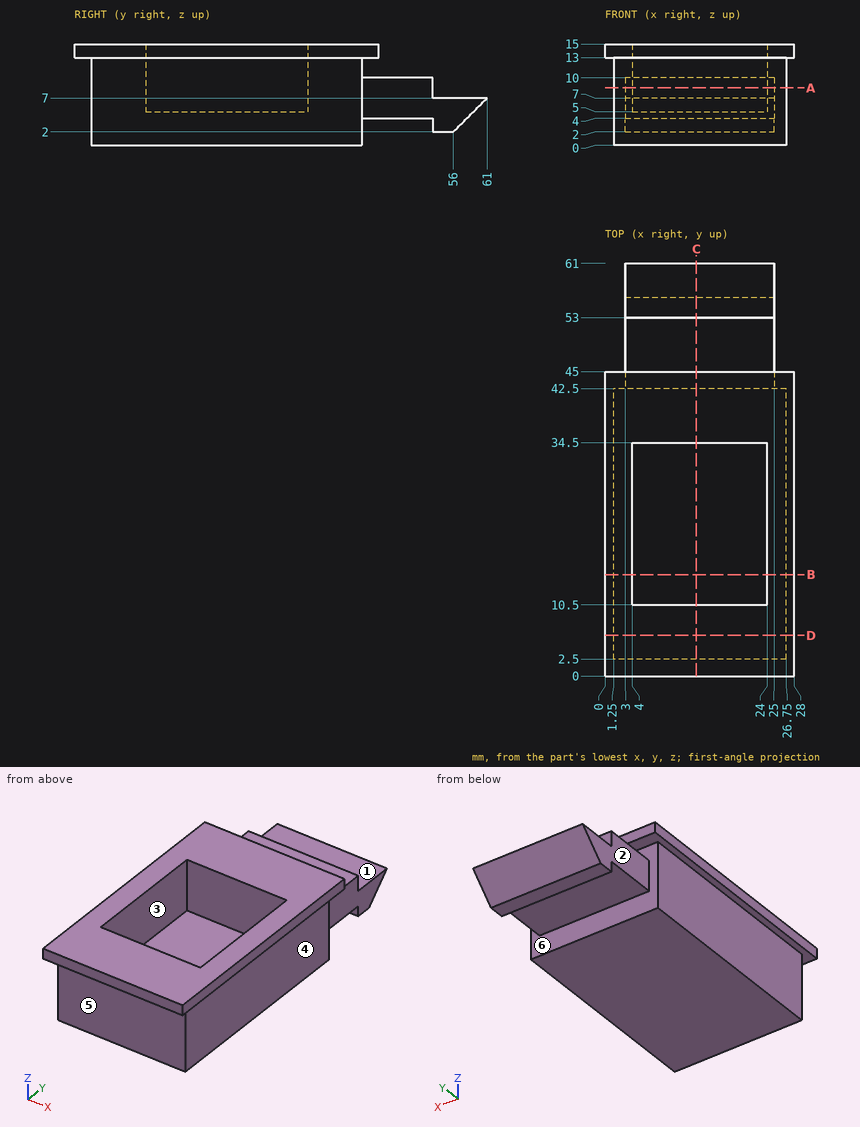
Geometry: see drawing. Coordinates: mm, zero at the bounding-box minimum. A direction names the side the tool comes from. Give positions to 0.01 mm unless a question says otherwise; leave off trailing zeros. Loops run counter-clockwise (first coordinate to the right, second up) from the corner with the lowest first, then second, coordinate; pieces in that order, holes last. Notation, with made-up numbers: M 12,-8.75 L 63,-8.75 A7 ccw 63,3.25 Z; hole C -32.5,-6 d7. An arc over 180 degrees is marked long. Answer as CSV lines item,"result". Start each with the question number.
1. Pin query (flat end, axial travel): P1, Ø1, axis at y = 9.5, z = 9, coming from the -X side; P2, Ø1.5, axis at x = 10.5, z = 9, coming from the +Y side; P3, Ø5, axis at y = 22.5, z = 12.5, coming from the +X side; P4, Ø1.6, axis at x = 18.5, z = 3.5, coming from the -Y side. Return the tip coordinate at first contact, or that it passes through.
2. Reachability of the marked faces 1, 2 and 3 from +Z, -Z, +X, -X, +Y, -Y: full face, straight path, thin tool, end or side. Return the list, or none.
3. Section D-D on y = 6. Return loops of the section in (x, z).
4. Section B-B on y = 15. Return loops of the section in (x, z).
5. Pull-direction query (Y, two-part tool) for the marked faces 4, 5 and 6; classes: released by +Y, released by -Y, zero draft, split by the parting line, or undercut.
6. Section C-C on x = 13.5. Return loops of the section in (y, z), plus the area to 4 significant figures.
7. Line query: L1, parallel to X at y = 13, z = 7.25; L2, parallel to Y at x = 19.75, z = 12; L3, parallel to Y at x = 2.25, z = 5.5. Output: solid intervals per line, ascending.
8. Section A-A on z = 8.5. Return loops of the section in (x, y).
Computed values:
1,P1,"stops at x = 1.25"
1,P2,"stops at y = 53"
1,P3,"stops at x = 28"
1,P4,"stops at y = 2.5"
2,face 1,"+Z, +X, -X, +Y"
2,face 2,"-Z, -X, +Y"
2,face 3,"+Z"
3,outline,"M 0,13 L 1.25,13 L 1.25,0 L 26.75,0 L 26.75,13 L 28,13 L 28,15 L 0,15 Z"
4,outline,"M 0,13 L 1.25,13 L 1.25,0 L 26.75,0 L 26.75,13 L 28,13 L 28,15 L 24,15 L 24,5 L 4,5 L 4,15 L 0,15 Z"
5,face 4,"zero draft"
5,face 5,"released by -Y"
5,face 6,"undercut"
6,outline,"M 0,13 L 2.5,13 L 2.5,0 L 42.5,0 L 42.5,4 L 53,4 L 53,2 L 56,2 L 61,7 L 53,7 L 53,10 L 42.5,10 L 42.5,13 L 45,13 L 45,15 L 34.5,15 L 34.5,5 L 10.5,5 L 10.5,15 L 0,15 Z"
6,area,"460.5 mm²"
7,L1,"x = 1.25 to 4, 24 to 26.75"
7,L2,"y = 2.5 to 10.5, 34.5 to 42.5"
7,L3,"y = 2.5 to 42.5"
8,outline,"M 1.25,2.5 L 26.75,2.5 L 26.75,42.5 L 25,42.5 L 25,53 L 3,53 L 3,42.5 L 1.25,42.5 Z; hole M 4,10.5 L 24,10.5 L 24,34.5 L 4,34.5 Z"
